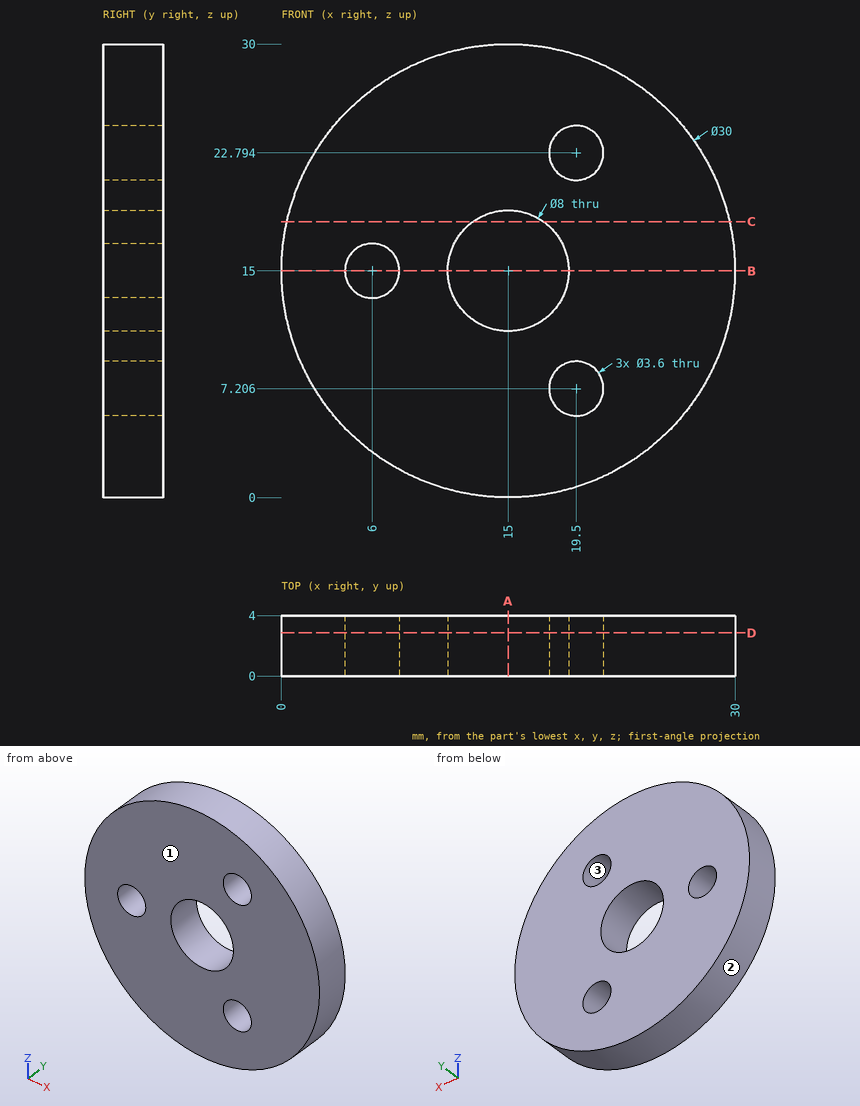
Part print with two shaded views. Sizes in mm from the minimum x, y, z corner. Give positions to 0.01 mm unless a question says otherwise; leave off trailing zeros. Order: outer loops, then holes, each group sorted by start corner. A loop starts at its lowest first (then second) coordinate and runs counter-clockwise, first axis right, second up.
(1) Saw through at D-D, the plane y = 2.85. Give the cut face in (x, z).
(2) Saw through at B-B, the plane z = 15. Give the cut face in (x, y).
(3) Saw through at A-A, the plane x = 15. Give the cut face in (y, z), then the cut area to 3 significant figures.
(4) Saw through at C-C, the plane z = 18.25. Give the cut face in (x, y).
(5) Drill centre lines: L1, parallel to Z at x = 20, y = 0.35 (1 decimal); L2, parallel to Z at x = 19.5, y = 1.65; L3, parallel to Z at x = 16.75, y = 0.35. Where is each one in solid material? Low to high.
(6) Mould opens along X. For the marked faces 1, 2 and 3 say: released by +X, released by -X, zero draft, split by the parting line, or undercut.
(7) Flat gauge pins, fed straight in: pin 1 (1.5 mm diameter, centred on y = 1, z = 21.5, fed in from +X); pin 2 (5 mm diameter, centred on x = 15, z = 15, fed in from +Y); pin 3 (2 mm diameter, centred on x = 24.5, y = 3, fed in from -Z). Where does each tip first touch, or does it go through?
Results found:
1. outline: circle Ø30 at (15, 15); hole circle Ø3.6 at (6, 15); hole circle Ø8 at (15, 15); hole circle Ø3.6 at (19.5, 7.21); hole circle Ø3.6 at (19.5, 22.79)
2. outline: (0, 0) - (4.2, 0) - (4.2, 4) - (0, 4) - close; (7.8, 0) - (11, 0) - (11, 4) - (7.8, 4) - close; (19, 0) - (30, 0) - (30, 4) - (19, 4) - close
3. outline: (0, 0) - (4, 0) - (4, 11) - (0, 11) - close; (0, 19) - (4, 19) - (4, 30) - (0, 30) - close
3. area: 88.0 mm2
4. outline: (0.36, 0) - (12.67, 0) - (12.67, 4) - (0.36, 4) - close; (17.33, 0) - (29.64, 0) - (29.64, 4) - (17.33, 4) - close
5. L1: z = 0.9 to 5.5, 8.9 to 21.1, 24.5 to 29.1
5. L2: z = 0.69 to 5.41, 9.01 to 20.99, 24.59 to 29.31
5. L3: z = 0.1 to 11.4, 18.6 to 29.9
6. face 1: zero draft
6. face 2: split by the parting line
6. face 3: undercut
7. pin 1: stops at x = 28.85
7. pin 2: passes through
7. pin 3: stops at z = 2.64
